Geometry check sheet. Reference: the model listing, model coordinates, mm. A direction names the side the tool comes from. Give positions to 0.01 mm unless a question says otherwise; leave off trailing zeros. Write each loop counter-clockwise with the first axis right and the second up, starting at its lowest first coordinate (ties: lowest second). Pieces come first, ordered by that corner, then holes.
(1) Depth check by flat-ended pin: P1, Ø12, axis at y = 3, z = 15, coming from the -X side; P2, Ø5, axis at x = 0, z = 9.5, coming from the +Y side; P3, Ø12, axis at y = 4.5, z = 12.5, coming from the +X side. Enter the tip coordinate at first touch or a pass-through.
(2) Cross-section at C-C (z = 9.75). Record the boundary of the cut face in (x, y).
(3) Cross-section at B-B (y = 4.5). Record the boundary of the cut face in (x, z), and give its area (3 significant figures).
(4) Cross-section at A-A (x = 0). Count the separate pieces of the cut face and the enclosed holes in it, and give its area (3 significant figures).
(5) Cross-section at D-D (y = 8.5). Record the boundary of the cut face in (x, z), and give its area (3 significant figures).
(6) Mould release check, pull along X, two halves, no side actions. Record for faces 1 (the flat face through (2, -2, 17)), 2 (the cylindrical face through (9.3, 7.6, 1.5)), 3 (the flat face through (0, 0, 0)): +X half, -X half, draft (parallel to the pull), parting line (faces both ways), or undercut.
(7) Tool access check on faces 4 (the flat face through (0, -0.75, 19)), 5 (the flat face through (6, 0, 3)), 6 (the flat face through (0, 9, 11)), 7 (the flat face through (-2, -2, 17)). Record the directions out of +Z, -Z, +X, -X, +Y, -Y that give a thin tool (end or side, any length) a straight path to the whole face; none if there is none.
(8) Thickness scan on line 1 along Y through (x, z) = (-10.5, 2.45); line 2 along X through (y, z) = (-6.2, 13); line 3 along X through (y, z) = (-5.75, 17.25). Record the ranges inside material, lowest first.
```python
from build123d import *

# Parameters (mm, degrees)
SKETCH1_W               = 27
SKETCH1_H               = 22
SKETCH1_R               = 1.5
BOSS_EXTRUDE1_DEPTH     = 3
SKETCH2_W               = 4
SKETCH2_H               = 18
BOSS_EXTRUDE2_DEPTH     = 18
CUT_EXTRUDE1_DEPTH      = 29.324018077
CUT_EXTRUDE1_DEPTH_BACK = 29.324018077
SKETCH3_R               = 4
CUT_EXTRUDE2_DEPTH      = 29.324018077
CUT_EXTRUDE2_DEPTH_BACK = 29.324018077
SKETCH4_W               = 8.09758535
SKETCH4_H               = 1.5
FILLET1_R               = 3
CUT_EXTRUDE3_DEPTH      = 34.275366264
CUT_EXTRUDE3_DEPTH_BACK = 34.275366264
SKETCH5_R               = 1.5
FILLET2_R               = 2
FILLET3_R               = 3


with BuildPart() as part:
    # Sketch1 → Boss-Extrude1 (new body)
    with BuildSketch(Plane.XY):
        Rectangle(SKETCH1_W, SKETCH1_H)
        with Locations((-10.5, -8.5)):
            Circle(SKETCH1_R, mode=Mode.SUBTRACT)
        with Locations((-10.5, 8.5)):
            Circle(SKETCH1_R, mode=Mode.SUBTRACT)
        with Locations((10.5, 8.5)):
            Circle(SKETCH1_R, mode=Mode.SUBTRACT)
        with Locations((10.5, -8.5)):
            Circle(SKETCH1_R, mode=Mode.SUBTRACT)
    extrude(amount=BOSS_EXTRUDE1_DEPTH)

    # Sketch2 → Boss-Extrude2 (add)
    with BuildSketch(Plane.XY.offset(3)):
        Rectangle(SKETCH2_W, SKETCH2_H)
    extrude(amount=BOSS_EXTRUDE2_DEPTH)

    # Sketch3 → Cut-Extrude1 (cut, two sides: drawn at the far end of the back side and taken through both)
    with BuildSketch(Plane(origin=(2, 0, 0), x_dir=(0, 0, -1), z_dir=(1, 0, 0)).offset(-CUT_EXTRUDE1_DEPTH_BACK)):
        with Locations(Location((-13, 0, 0), (0, 0, 180))):
            Circle(SKETCH3_R)
    extrude(amount=CUT_EXTRUDE1_DEPTH + CUT_EXTRUDE1_DEPTH_BACK, mode=Mode.SUBTRACT)

    # Sketch4 → Cut-Extrude2 (cut, two sides: drawn at the far end of the back side and taken through both)
    with BuildSketch(Plane(origin=(2, 0, 0), x_dir=(0, 0, -1), z_dir=(1, 0, 0)).offset(-CUT_EXTRUDE2_DEPTH_BACK)):
        with Locations((-18.330812417, 0)):
            Rectangle(SKETCH4_W, SKETCH4_H)
    extrude(amount=CUT_EXTRUDE2_DEPTH + CUT_EXTRUDE2_DEPTH_BACK, mode=Mode.SUBTRACT)

    # Fillet1
    fillet1_edges = [part.edges().sort_by_distance(p)[0] for p in [
        (-2, 0, 3),
        (2, 0, 3),
    ]]
    fillet(fillet1_edges, radius=FILLET1_R)

    # Sketch5 → Cut-Extrude3 (cut, two sides: drawn at the far end of the back side and taken through both)
    with BuildSketch(Plane(origin=(0, 11, 0), x_dir=(1, 0, 0), z_dir=(0, 1, 0)).offset(-CUT_EXTRUDE3_DEPTH_BACK)):
        with Locations(Location((0, -13, 0), (0, 0, 270))):
            Circle(SKETCH5_R)
    extrude(amount=CUT_EXTRUDE3_DEPTH + CUT_EXTRUDE3_DEPTH_BACK, mode=Mode.SUBTRACT)

    # Fillet2
    fillet2_edges = [part.edges().sort_by_distance(p)[0] for p in [
        (0, -9, 3),
        (0, 9, 3),
    ]]
    fillet(fillet2_edges, radius=FILLET2_R - 0.0001)  # a hair under: the kernel refuses the full size

    # Fillet3
    fillet3_edges = [part.edges().sort_by_distance(p)[0] for p in [
        (0, -9, 21),
        (0, 9, 21),
    ]]
    fillet(fillet3_edges, radius=FILLET3_R)


solid = part.part
```
Reply:
1. P1: stops at x = -2
1. P2: stops at y = 9
1. P3: stops at x = 2
2. outline: (-2, -9) - (2, -9) - (2, -2.33) - (-2, -2.33) - close; (-2, 2.33) - (2, 2.33) - (2, 9) - (-2, 9) - close
3. outline: (-13.5, 0) - (13.5, 0) - (13.5, 3) - (5, 3) arc R3 cw to (2, 6) - (2, 21) - (-2, 21) - (-2, 6) arc R3 cw to (-5, 3) - (-13.5, 3) - close; hole circle Ø3 at (0, 13)
3. area: 150 mm2
4. separate pieces: 3
4. enclosed holes: 0
4. area: 301 mm2
5. outline: (-13.5, 0) - (-12, 0) - (-12, 3) - (-13.5, 3) - close; (-9, 0) - (9, 0) - (9, 3) - (5, 3) arc R3 cw to (2, 6) - (2, 19.66) - (-2, 19.66) - (-2, 6) arc R3 cw to (-5, 3) - (-9, 3) - close; (12, 0) - (13.5, 0) - (13.5, 3) - (12, 3) - close; hole circle Ø3 at (0, 13)
5. area: 126 mm2
6. face 1: +X half
6. face 2: undercut
6. face 3: draft
7. face 4: +Z, +X, -X
7. face 5: +Z, +Y, -Y
7. face 6: +Z, +X, -X, +Y
7. face 7: +Z, -X, +Y, -Y
8. line 1: y = -11 to -10, -7 to 7, 10 to 11
8. line 2: x = -2 to -1.5, 1.5 to 2
8. line 3: x = -2 to 2
